Design review of the part shown in the three views and the two pictorial views. Dimensions are in mm from the part's minimum x, y and z. A direction names the side the tool comes from. Round coordinates to 2 decimals unless told otherwise and drop trailing zeros. Loops run counter-clockwise (first coordinate to the right, second up) from the corner with the lowest first, then second, coordinate; pieces in that order, holes last. Notation, with made-up numbers: (54.5, -37) -> (89.5, -37) arc R6 cw to (89.5, -30) -> close; hole circle Ø11 at (-11.75, -11). An arc over 180 degrees is marked (long way). One line per question, with ' | ' between items. Start each with the question number.
1. Consider section A-A (x = 25). Write out the cut boundary in (y, z).
2. For the marked faces 1, 2 and 3, list the 3-axis set-ups (+Z, -Z, +X, -X, +Y, -Y) from which the entire face can be reached by the end or side of a thin tool; tool diameter is ignored.
3. Wall thickness on line 1 along Y through (x, z) = (3.75, 7.5); line 2 along Y through (x, z) = (23.5, 2); line 3 along Y through (x, z) = (8, 1): over which ranges is each line inside the solid? List them lowest first.
4. Consider section D-D (x = 4). Write out the cut boundary in (y, z), and give its area (3 significant figures).
5. Consider section C-C (y = 6). Write out the cut boundary in (x, z).
6. Consider section B-B (z = 7.5). Write out the cut boundary in (x, y), and give its area (3 significant figures).
7. For pin 1 Ø3 at (x, y) = (30.5, 8.5) entering from -Z; pin 2 Ø4.5 at (x, z) = (28, 4) entering from +Y; pin 3 Ø5 at (x, z) = (5, 3.5) entering from -Y; pin 4 Ø6 at (y, z) = (18.5, 7.5) entering from +X, all flat-tipped, find the tip position at first contact; note any pin that passes through.
8. Draft analysis for pull direction Z (two halves, no side actions). For the marked faces 4, 5, 6 and 7, state which applies: pulls with the +Z half, pulls with the -Z half, needs draft (parallel to the pull), parting line crosses it, or undercut.
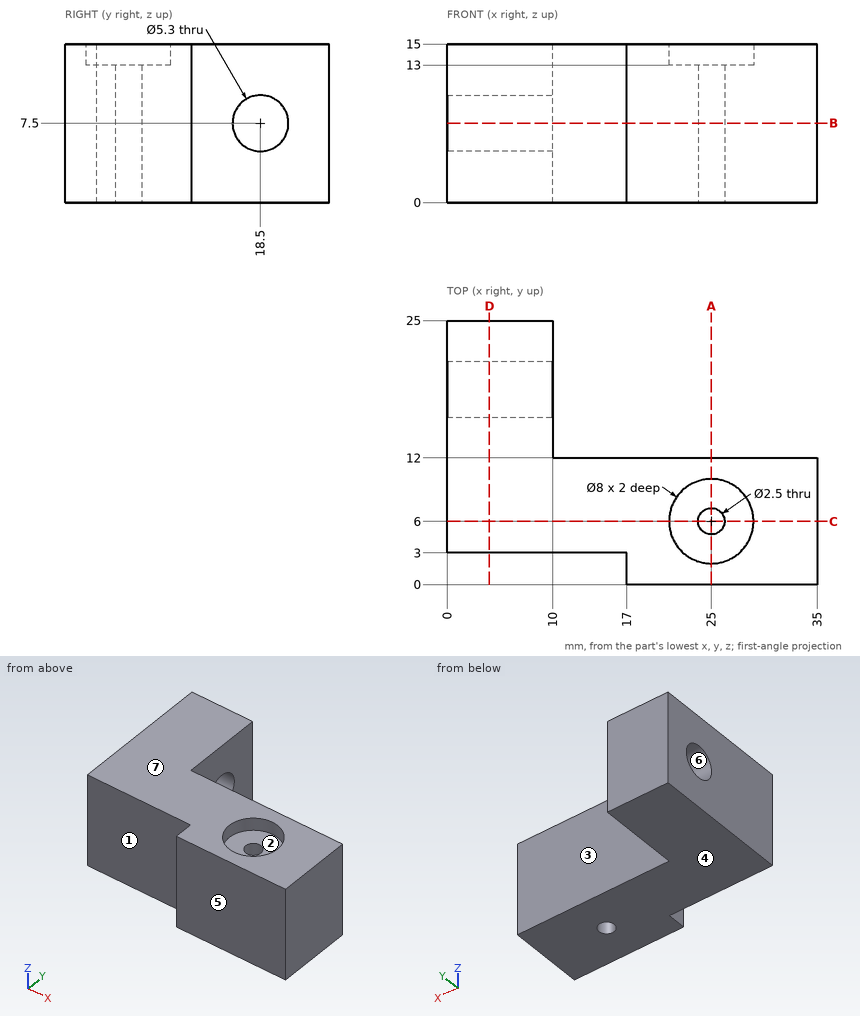
Answer block:
1) outline: (0, 0) -> (4.75, 0) -> (4.75, 13) -> (2, 13) -> (2, 15) -> (0, 15) -> close; (7.25, 0) -> (12, 0) -> (12, 15) -> (10, 15) -> (10, 13) -> (7.25, 13) -> close
2) face 1: +Z, -Z, -X, -Y | face 2: +Z | face 3: +Z, -Z, +X, +Y
3) line 1: y = 3 to 15.85, 21.15 to 25 | line 2: y = 0 to 12 | line 3: y = 3 to 25
4) outline: (3, 0) -> (25, 0) -> (25, 15) -> (3, 15) -> close; hole circle Ø5.3 at (18.5, 7.5) | area: 308 mm2
5) outline: (0, 0) -> (23.75, 0) -> (23.75, 13) -> (21, 13) -> (21, 15) -> (0, 15) -> close; (26.25, 0) -> (35, 0) -> (35, 15) -> (29, 15) -> (29, 13) -> (26.25, 13) -> close
6) outline: (0, 3) -> (17, 3) -> (17, 0) -> (35, 0) -> (35, 12) -> (10, 12) -> (10, 15.85) -> (0, 15.85) -> close; (0, 21.15) -> (10, 21.15) -> (10, 25) -> (0, 25) -> close; hole circle Ø2.5 at (25, 6) | area: 441 mm2
7) pin 1: stops at z = 0 | pin 2: stops at y = 12 | pin 3: stops at y = 3 | pin 4: stops at x = 10
8) face 4: pulls with the -Z half | face 5: needs draft | face 6: undercut | face 7: pulls with the +Z half
